```python
from build123d import *

# Parameters (mm, degrees)
SKETCH_4_W           = 84.916455131
SKETCH_4_H           = 80
SKETCH_4_R           = 3
EXTRUDE_1_DEPTH      = 7
EXTRUDE_2_DEPTH      = 3
EXTRUDE_2_DEPTH_BACK = 7
SKETCH_5_R           = 3
SKETCH_6_W           = 78
SKETCH_6_H           = 4.15
CUT_EXTRUDE_1_DEPTH  = 5
CUT_EXTRUDE_2_DEPTH  = 1
SKETCH_8_R           = 4.15
CUT_EXTRUDE_3_DEPTH  = 108.873135035


with BuildPart() as part:
    # 草图4 → 凸台-拉伸1 (new body)
    with BuildSketch(Plane(origin=(0, 0, 0), x_dir=(1, 0, 0), z_dir=(0, 1, 0))):
        with Locations((-1.967483917, -58.11712094)):
            Rectangle(SKETCH_4_W, SKETCH_4_H)
        with Locations(Location((-36.585071707, -25.636349073, 0), (0, 0, 270))):
            Circle(SKETCH_4_R, mode=Mode.SUBTRACT)
        with Locations(Location((32.601613083, -25.636349073, 0), (0, 0, 270))):
            Circle(SKETCH_4_R, mode=Mode.SUBTRACT)
        with Locations(Location((-36.585071707, -90.861964123, 0), (0, 0, 270))):
            Circle(SKETCH_4_R, mode=Mode.SUBTRACT)
        with Locations(Location((32.601613083, -90.861964123, 0), (0, 0, 270))):
            Circle(SKETCH_4_R, mode=Mode.SUBTRACT)
    extrude(amount=EXTRUDE_1_DEPTH)

    # 草图5 → 凸台-拉伸2 (add, two sides: drawn at the far end of the back side and taken through both)
    with BuildSketch(Plane(origin=(0, 7, 0), x_dir=(1, 0, 0), z_dir=(0, 1, 0)).offset(-EXTRUDE_2_DEPTH_BACK)):
        with Locations(Location((-36.585071707, -25.636349073, 0), (0, 0, 270))):
            Circle(SKETCH_5_R)
        with Locations(Location((32.601613083, -25.636349073, 0), (0, 0, 270))):
            Circle(SKETCH_5_R)
        with Locations(Location((-36.585071707, -90.861964123, 0), (0, 0, 270))):
            Circle(SKETCH_5_R)
        with Locations(Location((32.601613083, -90.861964123, 0), (0, 0, 270))):
            Circle(SKETCH_5_R)
    extrude(amount=EXTRUDE_2_DEPTH + EXTRUDE_2_DEPTH_BACK)

    # 草图6 → 切除-拉伸1 (cut)
    with BuildSketch(Plane.XZ):
        with Locations((-1.967483917, 60.19212094)):
            Rectangle(SKETCH_6_W, SKETCH_6_H)
        with Locations((-1.967483917, 56.04212094)):
            Rectangle(SKETCH_6_W, SKETCH_6_H)
    extrude(amount=-CUT_EXTRUDE_1_DEPTH, mode=Mode.SUBTRACT)

    # 草图7 → 切除-拉伸2 (cut)
    with BuildSketch(Plane.XZ.offset(-5)):
        with BuildLine():
            add(Edge.make_bspline(
                [(37.032516083, 58.11712094), (37.032516083, 62.26712094), (-1.967483917, 62.26712094), (-40.967483917, 62.26712094), (-40.967483917, 58.11712094)],
                knots=[3.141592654, 3.141592654, 3.141592654, 4.71238898, 4.71238898, 6.283185307, 6.283185307, 6.283185307], degree=2, weights=[1, 0.707106781, 1, 0.707106781, 1]))
            Line((-40.967483917, 58.11712094), (37.032516083, 58.11712094))
        make_face()
        with BuildLine():
            Line((37.032516083, 58.11712094), (-40.967483917, 58.11712094))
            add(Edge.make_bspline(
                [(-40.967483917, 58.11712094), (-40.967483917, 53.96712094), (-1.967483917, 53.96712094), (37.032516083, 53.96712094), (37.032516083, 58.11712094)],
                knots=[0, 0, 0, 1.570796327, 1.570796327, 3.141592654, 3.141592654, 3.141592654], degree=2, weights=[1, 0.707106781, 1, 0.707106781, 1]))
        make_face()
    extrude(amount=-CUT_EXTRUDE_2_DEPTH, mode=Mode.SUBTRACT)

    # 草图8 → 切除-拉伸3 (cut, through all)
    with BuildSketch(Plane.XZ.offset(-6)):
        with Locations(Location((-1.967483917, 58.11712094, 0), (0, 0, 270))):
            Circle(SKETCH_8_R)
    extrude(amount=-CUT_EXTRUDE_3_DEPTH, mode=Mode.SUBTRACT)


solid = part.part
```
For this review, take the finished solid that the model builds, in its own axes (mm). A direction names the side the tool comes from. Round coordinates to 2 decimals unless told otherwise and drop trailing zeros. Order: outer loops, then holes, each group sorted by start corner. A loop starts at its lowest first (then second) coordinate and runs counter-clockwise, first axis right, second up.
Q1. Machinability: for faces 1 (the cylindrical face through (35.13, 8.48, 27.25)), 2 (the flat face through (37.033, 2, 58)), 3 (the flat face through (-37, 10, 26)), which of the approach directions +Z, -Z, +X, -X, +Y, -Y give a long, thin tool a straight path to every point of the face, cutting with its end or side? Answer none if there is none.
Findings below:
face 1: +Y
face 2: -Y
face 3: +Z, -Z, +X, -X, +Y
Q2. We need section D-D, the plane z = 26. Give the boundary of the cut face in (x, y).
Findings below:
outline: (-44.43, 0) - (40.49, 0) - (40.49, 7) - (35.58, 7) - (35.58, 10) - (29.62, 10) - (29.62, 7) - (-33.61, 7) - (-33.61, 10) - (-39.56, 10) - (-39.56, 7) - (-44.43, 7) - close
Q3. Insertion check: P1, Ø4, axis at x = 10.5, z = 56, coming from the -Y side; P2, Ø10, axis at x = -22, z = 30.5, coming from the +Y side; P3, Ø4, axis at x = -30, z = 58.5, coming from the -Y side; P4, Ø1, axis at x = -5, y = 8.5, coming from the +Z side. Each pin has a flat end and moves straight along its axis. Give the tip position at first contact, or say it passes through.
Findings below:
P1: stops at y = 5
P2: stops at y = 7
P3: stops at y = 6
P4: passes through
Q4. Mouldability with a two-part tool opening along Z and no side actions: class faces 4 (the flat face through (29, 5, 55)), 5 (the cylindrical face through (34.63, 8.48, 88.65)), 6 (the flat face through (40.491, 3, 59)), 7 (the flat face through (-3, 3, 18.117)) as pulls with the +Z half, pulls with the -Z half, needs draft (parallel to the pull), parting line crosses it, or undercut.
Findings below:
face 4: undercut
face 5: undercut
face 6: needs draft
face 7: pulls with the -Z half
Q5. We need section A-A, the plane y = 1. Give the boundary of the cut face in (x, z).
Findings below:
outline: (-44.43, 18.12) - (40.49, 18.12) - (40.49, 98.12) - (-44.43, 98.12) - close; hole (-40.97, 53.97) - (37.03, 53.97) - (37.03, 62.27) - (-40.97, 62.27) - close
Q6. Wall thickness on line 1 (Z direction, x = -10.5, y = 1.5); line 2 (X direction, y = 9, z = 26); line 3 (Y direction, x = 3.5, z = 80): over which ranges is each line inside the solid? List them lowest first.
Findings below:
line 1: z = 18.12 to 53.97, 62.27 to 98.12
line 2: x = -39.56 to -33.61, 29.62 to 35.58
line 3: y = 0 to 7
Q7. We need section C-C, the plane y = 8.5. Give the boundary of the cut face in (x, z).
Findings below:
outline: circle Ø6 at (-36.59, 25.64); circle Ø6 at (-36.59, 90.86); circle Ø6 at (32.6, 25.64); circle Ø6 at (32.6, 90.86)
Q8. We need section B-B, the plane z = 86.5. Give the boundary of the cut face in (x, y), plus the area to 3 significant figures.
Findings below:
outline: (-44.43, 0) - (40.49, 0) - (40.49, 7) - (-44.43, 7) - close
area: 594 mm2
